Design review of the part built by this model. Coordinates are the model's own, in mm. A direction names the side the tool comes from. Coordinates: 2 decimals unless noted, no trailing zeros. Loops run counter-clockwise (first coordinate to the right, second up) from the corner with the lowest first, then second, coordinate; pieces in that order, holes last. Notation, with made-up numbers: (55, -20.75) -> (69, -20.75) arc R19 cw to (69, -16.75) -> close; hole circle Ø10 at (86, 61.25). An arc over 180 degrees is marked (long way). Use a Markdown table: item, result. Add a question column.
Q1. Take a section at A-A on y = 0. Write out the cut boundary in (x, z).
Q2. For faces 4 (the face through (0, 0, 0)), 5 (the face through (0, -29, 80)), list the 3-axis set-ups (+Z, -Z, +X, -X, +Y, -Y) from which the entire face can be reached by the end or side of a thin tool; tool diameter is ignored.
Q3. Draft analysis for pull direction Y (two halves, no side actions). For faces 1 (the face through (-0.52, -5.59, 87.35)), 2 (the face through (23.434, 7.38, 39.496)), 3 (the face through (0, 29, 80)), state which applies: pulls with the +Y half, pulls with the -Y half, needs draft (parallel to the pull), parting line crosses it, or undercut.
Q4. Take a section at D-D on z = 74.5. Write out the cut boundary in (x, y), plus the area to 3 significant figures.
Q5. For probe 1 along Z at (x, y) = (-10.5, 0); probe 2 along Z at (x, y) = (15, 26.5); probe 3 along Z at (x, y) = (17.5, 10.5), list the stretches that pass through material, from the lowest coordinate up.
Q6. Clearance check with flat-ended pins moving along their axes: pin 1 Ø10 at (y, z) = (1, 55.5) entering from -X; pin 2 Ø10 at (x, y) = (-18, 27.5) entering from -Z; pin 3 Ø20.5 at (x, y) = (2, -26) entering from -Z; pin 4 Ø10 at (x, y) = (-23, 29) entering from -Z. State where each tip first meets the part, or that it passes through.
Q7. Take a section at C-C on z = 19. Write out the cut boundary in (x, y).
Q8. Take a section at B-B on x = 0. Write out the cut boundary in (y, z).
from build123d import *

# Parameters (mm, degrees)
SKETCH1_R               = 24.568302704
EXTRUDE1_DEPTH          = 80
SKETCH2_R               = 37.339605778
EXTRUDE2_DEPTH          = 32
FILLET1_R               = 4
CUT_EXTRUDE1_DEPTH      = 32
CUT_EXTRUDE1_DEPTH_BACK = 77
SKETCH3_R               = 16.855421097


with BuildPart() as part:
    # Sketch1 → Extrude1 (new body)
    with BuildSketch(Plane.XY):
        Circle(SKETCH1_R)
    extrude(amount=EXTRUDE1_DEPTH)

    # Sketch2 → Extrude2 (add)
    with BuildSketch(Plane.XY.offset(80)):
        Circle(SKETCH2_R)
    extrude(amount=EXTRUDE2_DEPTH)

    # Fillet1
    fillet1_edges = [part.edges().sort_by_distance(p)[0] for p in [
        (-24.568302704, 0, 0),
        (-24.568302704, 0, 80),
        (-37.339605778, 0, 80),
        (-37.339605778, 0, 112),
    ]]
    fillet(fillet1_edges, radius=FILLET1_R)

    # Sketch3 → Cut-Extrude1 (cut, two sides: drawn at the far end of the back side and taken through both)
    with BuildSketch(Plane(origin=(25, 0, 0), x_dir=(0, 0, -1), z_dir=(1, 0, 0)).offset(-CUT_EXTRUDE1_DEPTH_BACK)):
        with Locations(Location((-71.449956272, 0, 0), (0, 0, 221.877807058))):
            Circle(SKETCH3_R)
    extrude(amount=CUT_EXTRUDE1_DEPTH + CUT_EXTRUDE1_DEPTH_BACK, mode=Mode.SUBTRACT)


solid = part.part
Answer list:
| question | item | result |
|---|---|---|
| 1 | outline | (-37.34, 88.31) -> (37.34, 88.31) -> (37.34, 108) arc R4 ccw to (33.34, 112) -> (-33.34, 112) arc R4 ccw to (-37.34, 108) -> close; (-24.57, 4) arc R4 ccw to (-20.57, 0) -> (20.57, 0) arc R4 ccw to (24.57, 4) -> (24.57, 54.59) -> (-24.57, 54.59) -> close |
| 2 | face 4 | -Z, +X, -X, +Y, -Y |
| 2 | face 5 | -Z, -Y |
| 3 | face 1 | undercut |
| 3 | face 2 | parting line crosses it |
| 3 | face 3 | needs draft |
| 4 | outline | (-18.13, -16.58) arc R24.57 ccw to (18.13, -16.58) -> close; (-18.13, 16.58) -> (18.13, 16.58) arc R24.57 ccw to start |
| 4 | area | 401 mm² |
| 5 | probe 1 | 0 to 54.59, 88.31 to 112 |
| 5 | probe 2 | 80 to 112 |
| 5 | probe 3 | 0 to 58.26, 84.64 to 112 |
| 6 | pin 1 | x = -24.57 |
| 6 | pin 2 | z = 79.94 |
| 6 | pin 3 | z = 0 |
| 6 | pin 4 | z = 80 |
| 7 | outline | circle Ø49.14 at (0, 0) |
| 8 | outline | (-37.34, 84) arc R4 ccw to (-33.34, 80) -> (-28.57, 80) arc R4 cw to (-24.57, 76) -> (-24.57, 4) arc R4 ccw to (-20.57, 0) -> (20.57, 0) arc R4 ccw to (24.57, 4) -> (24.57, 76) arc R4 cw to (28.57, 80) -> (33.34, 80) arc R4 ccw to (37.34, 84) -> (37.34, 108) arc R4 ccw to (33.34, 112) -> (-33.34, 112) arc R4 ccw to (-37.34, 108) -> close; hole circle Ø33.71 at (0, 71.45) |
